Part model, mm, in its own coordinate system. Round coordinates to 2 decimals unless told otherwise and drop trailing zeros. Loops run counter-clockwise (first coordinate to the right, second up) from the corner with the lowest first, then second, coordinate; pieces in that order, holes last. Notation, with made-up numbers: (70.5, -14.75) -> (120.5, -14.75) arc R29 cw to (120.5, 18.25) -> close; hole circle Ø1 at (39, 33.25). An arc over 180 degrees is marked (long way). Answer as CSV lines item,"result".
from build123d import *

# Parameters (mm, degrees)
SKETCH1_R           = 1.35
SKETCH1_R_2         = 0.875
SKETCH1_R_3         = 0.8001
BOSS_EXTRUDE1_DEPTH = 1.5875


with BuildPart() as part:
    # Sketch1 → Boss-Extrude1 (new body)
    with BuildSketch(Plane(origin=(0, 0, 0), x_dir=(1, 0, 0), z_dir=(0, 1, 0))):
        Polygon((22.5, 0), (23, 0.5), (23, 41.5), (22.5, 42), (20.25, 42), (19.75, 41.5), (13.75, 41.5), (13.25, 42), (9.75, 42), (9.25, 41.5), (3.25, 41.5), (2.75, 42), (0.5, 42), (0, 41.5), (0, 0.5), (0.5, 0), align=None)
        with Locations((12.36, 16.96)):
            Circle(SKETCH1_R, mode=Mode.SUBTRACT)
        with Locations((16.36, 16.96)):
            Circle(SKETCH1_R, mode=Mode.SUBTRACT)
        with Locations((12.36, 20.96)):
            Circle(SKETCH1_R, mode=Mode.SUBTRACT)
        with Locations((16.36, 20.96)):
            Circle(SKETCH1_R, mode=Mode.SUBTRACT)
        with Locations((12.36, 24.96)):
            Circle(SKETCH1_R, mode=Mode.SUBTRACT)
        with Locations((16.36, 24.96)):
            Circle(SKETCH1_R, mode=Mode.SUBTRACT)
        with Locations((21.5, 40)):
            Circle(SKETCH1_R_2, mode=Mode.SUBTRACT)
        with Locations((21.5, 2)):
            Circle(SKETCH1_R_2, mode=Mode.SUBTRACT)
        with Locations((1.5, 2)):
            Circle(SKETCH1_R_2, mode=Mode.SUBTRACT)
        with Locations((1.5, 40)):
            Circle(SKETCH1_R_2, mode=Mode.SUBTRACT)
        with Locations((11.5154, 40.2552)):
            Circle(SKETCH1_R_3, mode=Mode.SUBTRACT)
    extrude(amount=BOSS_EXTRUDE1_DEPTH)


solid = part.part
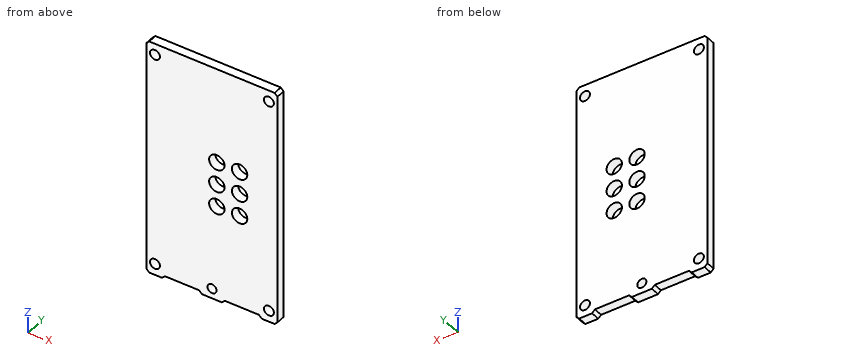
Q1. Saw through at B-B, the plane z = -16.96. Write the cut outline in (x, y).
Geometry results:
outline,"(0, 0) -> (11.01, 0) -> (11.01, 1.59) -> (0, 1.59) -> close; (13.71, 0) -> (15.01, 0) -> (15.01, 1.59) -> (13.71, 1.59) -> close; (17.71, 0) -> (23, 0) -> (23, 1.59) -> (17.71, 1.59) -> close"
Q2. Saw through at C-C, the plane y = 1.2. Give the number of separate pieces and of enclosed holes in the cut face, then the cut area to 3 significant figures.
Geometry results:
separate pieces,"1"
enclosed holes,"11"
area,"913 mm2"
Q3. Drop a flat-ended pin along its axis: P1, Ø0.8, axis at x = 7, y = 1, coming from the -Z side. Give the stop position or say it passes through.
Geometry results:
P1,"z = -41.5"
Q4. Drill centre lines: line 1 along X through (y, z) = (0.85, -20.96); line 2 along X through (y, z) = (0.5, -2) (3 decimals); line 3 along Z through (x, y) = (16.25, 0.15). Where is each one in solid material? Low to high.
Geometry results:
line 1,"0 to 11.01, 13.71 to 15.01, 17.71 to 23"
line 2,"0 to 0.625, 2.375 to 20.625, 22.375 to 23"
line 3,"-41.5 to -26.31, -23.61 to -22.31, -19.61 to -18.31, -15.61 to 0"
Q5. Saw through at A-A, the plane x = 21.5. Write the cut outline in (y, z) (1 decimal).
Geometry results:
outline,"(0, -42) -> (1.6, -42) -> (1.6, -40.9) -> (0, -40.9) -> close; (0, -39.1) -> (1.6, -39.1) -> (1.6, -2.9) -> (0, -2.9) -> close; (0, -1.1) -> (1.6, -1.1) -> (1.6, 0) -> (0, 0) -> close"
